The model under review builds one solid part; all positions refer to its coordinate system, in mm. A direction names the side the tool comes from. Coordinates: 2 decimals unless noted, no trailing zeros. Loops run counter-clockwise (first coordinate to the right, second up) from the corner with the lowest first, then second, coordinate; pieces in that order, holes last. Notation, with made-up numbers: M 15,9.25 L 22,9.25 A22 cw 22,32.25 Z; hole C -33,2 d6. An arc over 180 degrees is marked long. One line per item, written item: value.
Autodesk Inventor part; units mm, degrees
ref_plane "YZ Plane" through (0, 0, 0) normal (1, 0, 0) x (0, 1, 0)
ref_plane "XZ Plane" through (0, 0, 0) normal (0, 1, 0) x (-1, 0, 0)
ref_plane "XY Plane" through (0, 0, 0) normal (0, 0, 1) x (1, 0, 0)
sketch "Sketch1" plane through (0, 0, 0) normal (0, 1, 0) x (-1, 0, 0)
  circle A0 centre (0, 0) radius 25
  dimension "d0" = 50
extrude "Extrusion1" add sketch "Sketch1" along normal blind 5
sketch "Sketch4" plane through (0, 5, 0) normal (0, 1, 0) x (1, 0, 0)
  circle A0 centre (0, 0) radius 20 construction
  circle A1 centre (0, -20) radius 2.5
  dimension "d8" = 40
  dimension "d9" = 5
extrude "Extrusion3" cut sketch "Sketch4" against normal through all
sketch "Sketch5" plane through (0, 0, 0) normal (0, -1, 0) x (1, 0, 0)
  circle A0 centre (0, 0) radius 10.5
  dimension "d12" = 21
extrude "Extrusion4" add sketch "Sketch5" along normal blind 3
sketch "Sketch6" plane through (0, -3, 0) normal (0, -1, 0) x (1, 0, 0)
  circle A0 centre (0, 0) radius 9.5
  dimension "d15" = 19
extrude "Extrusion5" add sketch "Sketch6" along normal blind 11
sketch "Sketch7" plane through (0, 5, 0) normal (0, 1, 0) x (1, 0, 0)
  circle A0 centre (0, 0) radius 7.5
  dimension "d18" = 15
extrude "Extrusion6" cut sketch "Sketch7" against normal blind 6
sketch "Sketch8" plane through (0, -1, 0) normal (0, 1, 0) x (1, 0, 0)
  circle A0 centre (0, 0) radius 3.5
  dimension "d21" = 7
extrude "Extrusion7" cut sketch "Sketch8" against normal through all
sketch "Sketch9" plane through (0, -14, 0) normal (0, -1, 0) x (1, 0, 0)
  circle A0 centre (0, 0) radius 3.5
  circle A1 centre (0, 0) radius 10.5
  circle A2 centre (0, 0) radius 7
  dimension "d24" = 14
extrude "Extrusion8" add sketch "Sketch9" along normal blind 5 contours A2
sketch "Sketch10" plane through (0, 0, 0) normal (0, -1, 0) x (1, 0, 0)
  line L0 (0, 0) -> (0, 39) construction
  circle A0 centre (0, 20) radius 2.5
properties part number "sprzeglo_03"
(1) Insertion check: pin 1 Ø4 at (y, z) = (1, 11) entering from +X; pin 2 Ø9 at (x, z) = (0, 0) entering from +Y; pin 3 Ø8 at (x, z) = (16.5, -18) entering from -Y. Each pin has a flat end and moves straight along its axis. Give the tip position at first contact, or say it passes through.
Checks:
pin 1: x = 23.32
pin 2: y = -1
pin 3: y = 0
(2) To check wall thickness, follow L1, parallel to Z at x = 0, y = 3.7; L2, parallel to Y at x = -8, z = -11; L3, parallel to Z at x = 0, y = -9.5. State the ranges of each line that lie inside material, in increasing order. Write a range as [from, to].
Checks:
L1: [-25, -7.5], [7.5, 17.5], [22.5, 25]
L2: [0, 5]
L3: [-9.5, -3.5], [3.5, 9.5]
(3) Add section D-D on z = 20. State the section outline as (x, y) points, then the cut area to 3 significant figures.
Checks:
outline: M -15,0 L -2.5,0 L -2.5,5 L -15,5 Z; M 2.5,0 L 15,0 L 15,5 L 2.5,5 Z
area: 125 mm^2
(4) Draft analysis for pull direction Z (two halves, no side actions). For faces 4 (the face through (-5, -3, -9)), 5 (the face through (10, -1.5, -3.2)), 6 (the face through (1.34, 2.54, 17.89)), state which applies: pulls with the +Z half, pulls with the -Z half, needs draft (parallel to the pull), parting line crosses it, or undercut.
Checks:
face 4: needs draft
face 5: parting line crosses it
face 6: undercut
(5) Tool access review of faces 1 (the face through (-4, -14, -6)), 2 (the face through (3.233, -9.874, 1.341)), 3 (the face through (-7.493, 2.042, -0.33)): name each direction out of +Z, -Z, +X, -X, +Y, -Y from which nothing blocks a thin tool from reaching the whole face with its end or side.
Checks:
face 1: -Y
face 2: +Y, -Y
face 3: +Y
(6) Add section B-B on z = 0. State the section outline as (x, y) points, then the cut area to 3 significant figures.
Checks:
outline: M -25,0 L -10.5,0 L -10.5,-3 L -9.5,-3 L -9.5,-14 L -7,-14 L -7,-19 L -3.5,-19 L -3.5,-1 L -7.5,-1 L -7.5,5 L -25,5 Z; M 3.5,-19 L 7,-19 L 7,-14 L 9.5,-14 L 9.5,-3 L 10.5,-3 L 10.5,0 L 25,0 L 25,5 L 7.5,5 L 7.5,-1 L 3.5,-1 Z
area: 376 mm^2
(7) Add section A-A on x = 0. State the section outline as (y, z) points.
Checks:
outline: M -19,-7 L -14,-7 L -14,-9.5 L -3,-9.5 L -3,-10.5 L 0,-10.5 L 0,-25 L 5,-25 L 5,-7.5 L -1,-7.5 L -1,-3.5 L -19,-3.5 Z; M -19,3.5 L -1,3.5 L -1,7.5 L 5,7.5 L 5,17.5 L 0,17.5 L 0,10.5 L -3,10.5 L -3,9.5 L -14,9.5 L -14,7 L -19,7 Z; M 0,22.5 L 5,22.5 L 5,25 L 0,25 Z
(8) Add section C-C on y = -17.5. State the section outline as (x, z) points.
Checks:
outline: C 0,0 d14; hole C 0,0 d7
